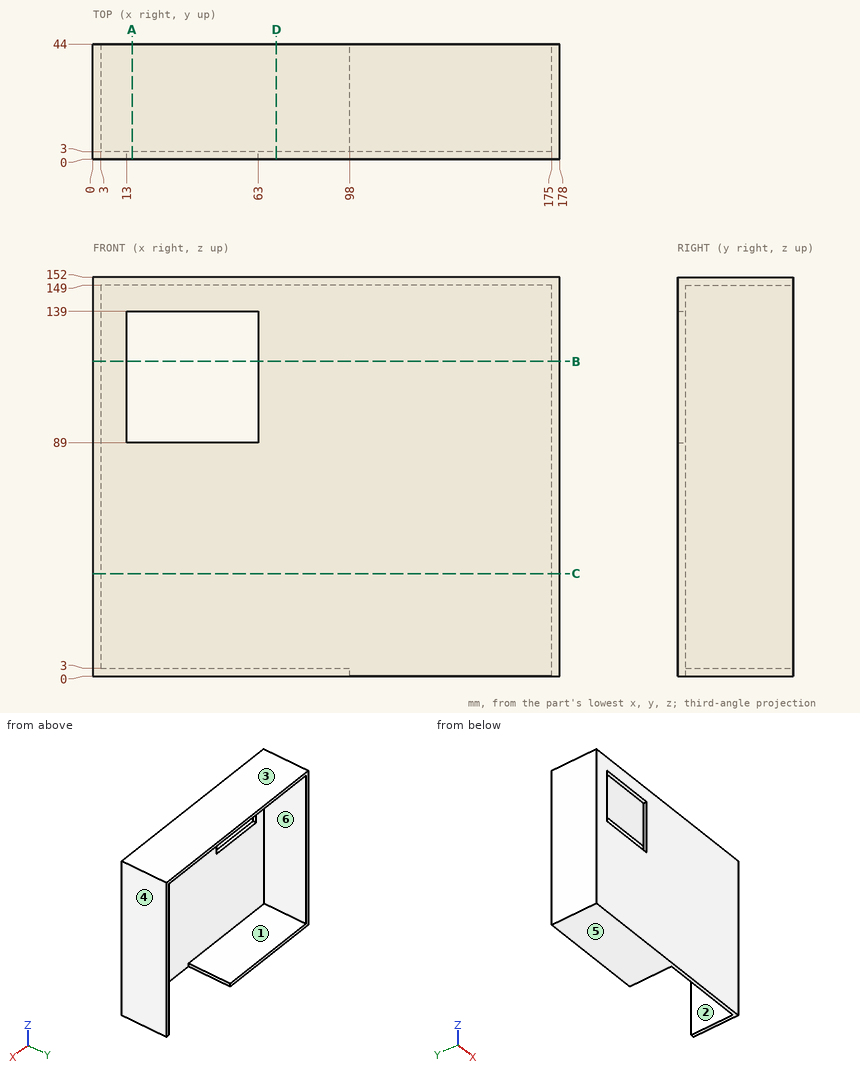
The figure shows three views and two pictorial views of one solid part (mm, origin at its lowest corner). Answer the questions. A direction names the side the tool comes from. Round coordinates to 2 decimals unless told otherwise and drop trailing zeros. Order: outer loops, then holes, each group sorted by start corner. A loop starts at its lowest first (then second) coordinate and runs counter-clockwise, first axis right, second up. Notation, with made-up numbers: (67, 89) - (124, 89) arc R21 cw to (124, 100) - close; hole circle Ø10 at (59, -11.75). An arc over 180 degrees is marked (long way). Write item = value, one per line. Start each with the question number.
1) For the marked faces 1, 2 and 3, determine the directions among +Z, -Z, +X, -X, +Y, -Y from which every point of the face is accessible in a straight line to the end or side of a thin tool.
2) Straight lines are drawn through the part: L1, parallel to Z at x = 88, y = 33; L2, parallel to X at y = 34, z = 100.5; L3, parallel to Z at x = 158.5, y = 28. For each, find the intervals that lie inside material, in ascending order.
3) Section A-A, the plane x = 15 is taken. Write down the section's boundary in (y, z), plus the area to 3 significant figures.
4) Section D-D, the plane x = 70 is taken. Write down the section's boundary in (y, z), plus the area to 3 significant figures.
5) Section B-B, the plane z = 120 is taken. Write down the section's boundary in (x, y).
6) Given pin 1 (12 mm diameter, centred on x = 154, y = 26.5, fed in from -Z), flat-ended and moving along its own axis, determine where the tip first touches the part or whether it passes through.
7) For a pull along X with two mould halves and no side action, classify the marked faces 4, 5 and 6 as released by +X, released by -X, zero draft, split by the parting line, or undercut.
8) Section C-C, the plane z = 39 is taken. Write down the section's boundary in (x, y), plus the area to 3 significant figures.
Results list:
q1.face_1 = +Y
q1.face_2 = -Z, +Y
q1.face_3 = +Z, +X, -X, +Y, -Y
q2.L1 = 0 to 3, 149 to 152
q2.L2 = 0 to 3, 175 to 178
q2.L3 = 149 to 152
q3.outline = (0, 0) - (44, 0) - (44, 3) - (3, 3) - (3, 89) - (0, 89) - close; (0, 139) - (3, 139) - (3, 149) - (44, 149) - (44, 152) - (0, 152) - close
q3.area = 552 mm^2
q4.outline = (0, 0) - (44, 0) - (44, 3) - (3, 3) - (3, 149) - (44, 149) - (44, 152) - (0, 152) - close
q4.area = 702 mm^2
q5.outline = (0, 0) - (13, 0) - (13, 3) - (3, 3) - (3, 44) - (0, 44) - close; (63, 0) - (178, 0) - (178, 44) - (175, 44) - (175, 3) - (63, 3) - close
q6.pin_1 = 149
q7.face_4 = released by +X
q7.face_5 = zero draft
q7.face_6 = undercut
q8.outline = (0, 0) - (178, 0) - (178, 44) - (175, 44) - (175, 3) - (3, 3) - (3, 44) - (0, 44) - close
q8.area = 780 mm^2
